Check sheet for the modelled part. Datum: model origin and axes. Units: mm. Face numbers are marked on the shaded views. A direction names the side the tool comes from. Coordinates: 2 decimals unless noted, no trailing zeros. Loops run counter-clockwise (first coordinate to the right, second up) from the corner with the lowest first, then second, coordinate; pieces in that order, holes last. Notation, with made-up numbers: (58, 74.25) -> (94, 74.25) arc R20 cw to (94, 86.25) -> close; hole circle Ø4 at (16.5, 49.5). An arc over 180 degrees is marked (long way). Use CSV: the item, a comma, the result in double quotes. Start each with the question number.
1. Sectioned sample at B-B, the plane y = 15.25. Record the cut outline in (x, z), and give its area (3 significant figures).
2. Sectioned sample at C-C, the plane z = 6.5. Record the cut outline in (x, y), and give its area (3 significant figures).
3. Sectioned sample at A-A, the plane x = 8. Record the cut outline in (y, z), and give its area (3 significant figures).
4. Set-up check for the marked faces 1 and 2: record each of +Z, -Z, +X, -X, +Y, -Y from which the full face is reachable in a straight line by a thin tool's end or side.
5. Sectioned sample at D-D, the plane x = 18.75. Record the cut outline in (y, z).
6. Thickness scan on L1, parallel to Y at x = 1, z = 0; L2, parallel to Y at x = 18.5, z = 7; L3, parallel to Z at x = 9.5, y = 1.25. Record the ranges inside material, lowest first.
7. Gauge pin test, flat ends, axial feed: pin 1 (4 mm diameter, centred on y = 18, z = 2.5, fed in from +X); pin 2 (1 mm diameter, centred on y = 22, z = -6, fed in from -X); pin 3 (5 mm diameter, centred on x = 15.5, z = 4.5, fed in from +Y). Record the tip position at first contact, or that the pin passes through.
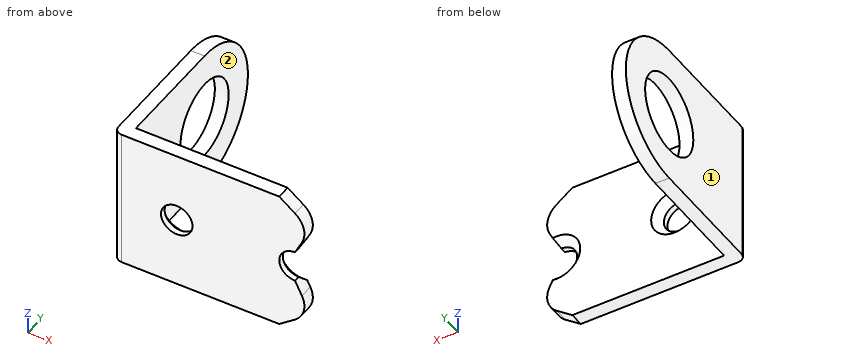
```python
from build123d import *

# Parameters (mm, degrees)
SKETCH_1_W          = 28
SKETCH_1_H          = 18
SKETCH_1_R          = 2
EXTRUDE_1_DEPTH     = 1.75
SKETCH_2_R          = 5
EXTRUDE_2_DEPTH     = 1.75
FILLET_1_R          = 1
CHAMFER_1_SIZE      = 1
CUT_EXTRUDE_1_REACH = 40.601


with BuildPart() as part:
    # Эскиз1 → Бобышка-Вытянуть1 (new body)
    with BuildSketch(Plane(origin=(0, 0, 0), x_dir=(1, 0, 0), z_dir=(0, 1, 0))):
        with Locations((14, 0)):
            Rectangle(SKETCH_1_W, SKETCH_1_H)
        with Locations(Location((8, 0, 0), (0, 0, 270))):
            Circle(SKETCH_1_R, mode=Mode.SUBTRACT)
        with Locations(Location((23, 0, 0), (0, 0, 270))):
            Circle(SKETCH_1_R, mode=Mode.SUBTRACT)
    extrude(amount=EXTRUDE_1_DEPTH)

    # Эскиз2 → Бобышка-Вытянуть2 (add)
    with BuildSketch(Plane(origin=(0, 0, 0), x_dir=(0, 0, -1), z_dir=(1, 0, 0))):
        with BuildLine():
            Line((-9, 0), (-9, 16))
            ThreePointArc((-9, 16), (0, 25), (9, 16))
            Line((9, 16), (9, 0))
            Line((9, 0), (-9, 0))
        make_face()
        with Locations((0, 16)):
            Circle(SKETCH_2_R, mode=Mode.SUBTRACT)
    extrude(amount=EXTRUDE_2_DEPTH)

    # Скругление1
    fillet_1_edges = [part.edges().sort_by_distance(p)[0] for p in [
        (0, 0, 0),
    ]]
    fillet(fillet_1_edges, radius=FILLET_1_R)

    # Фаска1
    chamfer_1_edges = [part.edges().sort_by_distance(p)[0] for p in [
        (8, 1.75, -2),
        (23, 1.75, -2),
    ]]
    chamfer(chamfer_1_edges, length=CHAMFER_1_SIZE)

    # Эскиз3 → Вырез-Вытянуть1 (cut, up to next)
    with BuildSketch(Plane(origin=(0, 0, 0), x_dir=(-1, 0, 0), z_dir=(0, -1, 0)), mode=Mode.PRIVATE) as cut_extrude_1_sk1:
        with BuildLine():
            ThreePointArc((-25, 0), (-24.414213562, 1.414213562), (-23, 2))
            Line((-23, 2), (-23.880298325, 3.76059665))
            ThreePointArc((-23.880298325, 3.76059665), (-24.11676372, 5.791496198), (-22.997016752, 7.502237436))
            Line((-22.997016752, 7.502237436), (-21, 9))
            Line((-21, 9), (-28, 9))
            Line((-28, 9), (-28, 0))
            Line((-28, 0), (-25, 0))
        make_face()
    cut_extrude_1_tool1 = extrude(cut_extrude_1_sk1.sketch, amount=-CUT_EXTRUDE_1_REACH, mode=Mode.PRIVATE) & part.part
    # Эскиз3 → Вырез-Вытянуть1 (cut, up to next)
    with BuildSketch(Plane(origin=(0, 0, 0), x_dir=(-1, 0, 0), z_dir=(0, -1, 0)), mode=Mode.PRIVATE) as cut_extrude_1_sk2:
        with BuildLine():
            ThreePointArc((-23, -2), (-24.414213562, -1.414213562), (-25, 0))
            Line((-25, 0), (-28, 0))
            Line((-28, 0), (-28, -9))
            Line((-28, -9), (-21, -9))
            Line((-21, -9), (-22.997016752, -7.502237436))
            ThreePointArc((-22.997016752, -7.502237436), (-24.11676372, -5.791496198), (-23.880298325, -3.76059665))
            Line((-23.880298325, -3.76059665), (-23, -2))
        make_face()
    cut_extrude_1_tool2 = extrude(cut_extrude_1_sk2.sketch, amount=-CUT_EXTRUDE_1_REACH, mode=Mode.PRIVATE) & part.part
    add(cut_extrude_1_tool1.solids().sort_by_distance((25.731211, 0, -4.895819))[0], mode=Mode.SUBTRACT)
    add(cut_extrude_1_tool2.solids().sort_by_distance((25.731211, 0, 4.895819))[0], mode=Mode.SUBTRACT)


solid = part.part
```
Completed:
1,outline,"(0, -9) -> (1.75, -9) -> (1.75, -4.94) -> (0, -4.94) -> close; (0, 4.94) -> (1.75, 4.94) -> (1.75, 9) -> (0, 9) -> close"
1,area,"14.2 mm²"
2,outline,"(0, 1) arc R1 ccw to (1, 0) -> (23.85, 0) -> (23.85, 1.75) -> (1.75, 1.75) -> (1.75, 22.22) -> (0, 22.22) -> close"
2,area,"77.4 mm²"
3,outline,"(0, -9) -> (1.75, -9) -> (1.75, -3) -> (0.75, -2) -> (0, -2) -> close; (0, 2) -> (0.75, 2) -> (1.75, 3) -> (1.75, 9) -> (0, 9) -> close"
3,area,"23.5 mm²"
4,face 1,"+Z, -Z, -X, +Y, -Y"
4,face 2,"+Z, -Z, +X, +Y"
5,outline,"(0, -9) -> (1.75, -9) -> (1.75, 9) -> (0, 9) -> close"
6,L1,"0 to 11, 21 to 25"
6,L2,"0 to 1.75"
6,L3,"-9 to -2, 2 to 9"
7,pin 1,"x = 1.75"
7,pin 2,"x = 0"
7,pin 3,"y = 1.75"
